Autodesk Inventor part; units mm, degrees
ref_plane "YZ Plane" through (0, 0, 0) normal (1, 0, 0) x (0, 1, 0)
ref_plane "XZ Plane" through (0, 0, 0) normal (0, 1, 0) x (-1, 0, 0)
ref_plane "XY Plane" through (0, 0, 0) normal (0, 0, 1) x (1, 0, 0)
sketch "Sketch1" plane through (0, 0, 0) normal (0, 1, 0) x (-1, 0, 0)
  line L0 (0, 0) -> (-100, 0)
  line L1 (-100, 0) -> (-100, -489)
  line L2 (-100, -489) -> (0, -489)
  line L3 (0, -489) -> (0, 0)
  dimension "d0" = 489
  dimension "d1" = 100
extrude "Extrusion1" add sketch "Sketch1" along normal blind 6.5
sketch "Sketch2" plane through (0, 6.5, 0) normal (0, 1, 0) x (1, 0, 0)
  line L0 (0, 489) -> (0, 0)
  line L1 (0, 459) -> (20, 439)
  line L2 (20, 439) -> (20, 65)
  line L3 (20, 65) -> (0, 45)
  line L4 (0, 459) -> (0, 45)
  dimension "d4" = 45
  dimension "d5" = 20
  dimension "d6" = 30
  dimension "d7" = 45
extrude "Extrusion2" cut sketch "Sketch2" against normal through all
properties part number "inner_brace_right"
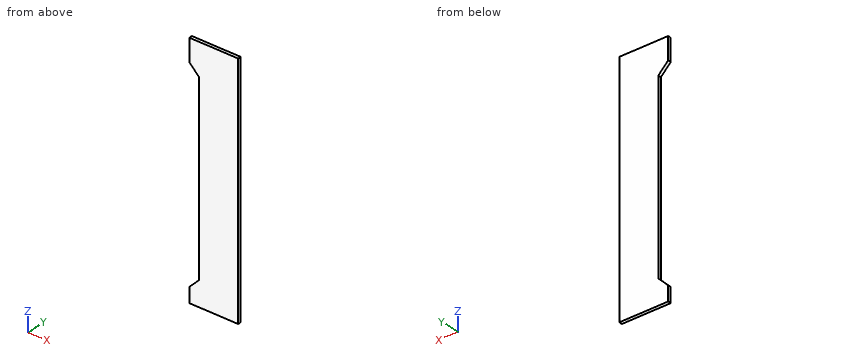
Geometry: final body of the model. Coordinates: model frame, mm. Coordinates: 2 decimals unless noted, no trailing zeros. Write each loop counter-clockwise with the first axis right and the second up, starting at its lowest first coordinate (ties: lowest second). Pieces come first, ordered by that corner, then holes. Notation, with made-up numbers: M 64,-32 L 95,-32 A26 ccw 95,5 Z; hole C 25.25,86 d7. An arc over 180 degrees is marked long. Answer as CSV lines item,"result". Start each with the question number.
Q1. Pin query (flat end, axial travel): P1, Ø3, axis at y = 4.5, z = -384.5, coming from the -X side; P2, Ø3, axis at x = 77, y = 1.5, coming from the +Z side. Return the tip coordinate at first contact, or that it passes through.
Q2. Line query: line 1 (X direction, y = 1.75, z = -366.5); line 2 (Z direction, x = 6, y = 2.75); line 3 (Z direction, x = 12, y = 4). Output: solid intervals per line, ascending. Write a range as from..to.
Q3. Cut plane B-B on z = -426. Return the cut outline in (x, y).
Q4. Cut plane A-A on y = 2.25. Return the cut outline in (x, z).
Findings below:
1,P1,"stops at x = 20"
1,P2,"stops at z = 0"
2,line 1,"x = 20..100"
2,line 2,"z = -489..-453, -51..0"
2,line 3,"z = -489..-447, -57..0"
3,outline,"M 20,0 L 100,0 L 100,6.5 L 20,6.5 Z"
4,outline,"M 0,-489 L 100,-489 L 100,0 L 0,0 L 0,-45 L 20,-65 L 20,-439 L 0,-459 Z"
